from build123d import *

# Parameters (mm, degrees)
F0_R     = 12.1
F0_R_2   = 3.25
F1_DEPTH = 10
F2_R     = 11
F2_R_2   = 3.25
F3_DEPTH = 9
F4_R     = 2
F5_R     = 2


with BuildPart() as f1:
    # F0 (on Top) → F1 (new body)
    with BuildSketch(Plane.XY):
        Circle(F0_R)
        Circle(F0_R_2, mode=Mode.SUBTRACT)
    extrude(amount=F1_DEPTH)

    # F2 (on face) → F3 (cut)
    with BuildSketch(Plane.XY.offset(10)):
        Circle(F2_R)
        Circle(F2_R_2, mode=Mode.SUBTRACT)
    extrude(amount=-F3_DEPTH, mode=Mode.SUBTRACT)

    # F4
    f4_edges = [f1.edges().sort_by_distance(p)[0] for p in [
        (-12.1, 0, 0),
    ]]
    fillet(f4_edges, radius=F4_R)

    # F5
    f5_edges = [f1.edges().sort_by_distance(p)[0] for p in [
        (-11, 0, 1),
    ]]
    fillet(f5_edges, radius=F5_R)


solid = f1.part
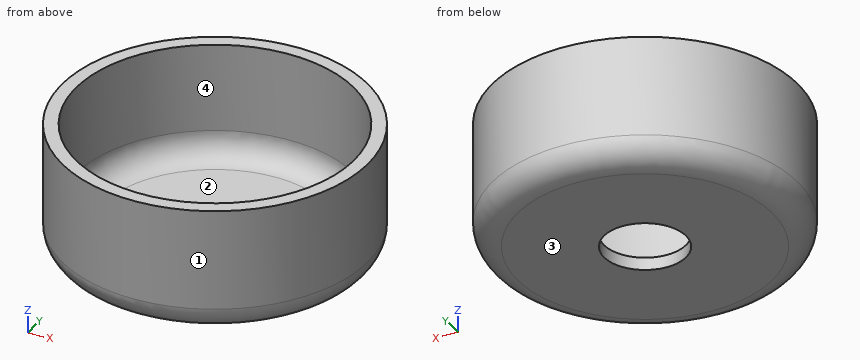
The model under review builds one solid part; all positions refer to its coordinate system, in mm. Face numbers are marked on the shaded views. Coordinates: 2 decimals unless noted, no trailing zeros. Loops run counter-clockwise (first coordinate to the right, second up) from the corner with the lowest first, then second, coordinate; pieces in that order, holes last. Notation, with made-up numbers: (-31.5, 65) -> (4.5, 65) arc R22 ccw to (4.5, 72) -> close; hole circle Ø7 at (32.5, -32.5). An arc over 180 degrees is marked (long way). Use a Markdown table: item, result. Add a question column.
1. Clearance check with flat-ended pins moving along their axes: pin 1 Ø9 at (x, y) = (-3, -1) entering from +Z; pin 2 Ø1.5 at (y, z) = (5, 4.5) entering from +X; pin 3 Ø3 at (x, z) = (8.5, 2) entering from +Y. State where each tip first meets the part, or that it passes through.
2. Add section C-C on z = 7.75. Write out the cut boundary in (x, y).
3. Draft analysis for pull direction X (two halves, no side actions). For the marked faces 1, 2, 3 and 4, state which applies: pulls with the +X half, pulls with the -X half, needs draft (parallel to the pull), parting line crosses it, or undercut.
4. Add section A-A on x = 0. Write out the cut boundary in (y, z).
5. To check wall thickness, follow line 1 (Y direction, x = 0, z = 8.75); line 2 (Z direction, x = 7.25, y = 1); line 3 (Y direction, x = 4.25, z = 7). State the ranges of each line that lie inside material, in increasing order.
Returned:
| question | item | result |
|---|---|---|
| 1 | pin 1 | stops at z = 1 |
| 1 | pin 2 | stops at x = 11.33 |
| 1 | pin 3 | stops at y = 9.87 |
| 2 | outline | circle Ø24.2 at (0, 0); hole circle Ø22 at (0, 0) |
| 3 | face 1 | parting line crosses it |
| 3 | face 2 | undercut |
| 3 | face 3 | needs draft |
| 3 | face 4 | undercut |
| 4 | outline | (-12.1, 2) arc R2 ccw to (-10.1, 0) -> (-3.25, 0) -> (-3.25, 1) -> (-9, 1) arc R2 cw to (-11, 3) -> (-11, 10) -> (-12.1, 10) -> close; (3.25, 0) -> (10.1, 0) arc R2 ccw to (12.1, 2) -> (12.1, 10) -> (11, 10) -> (11, 3) arc R2 cw to (9, 1) -> (3.25, 1) -> close |
| 5 | line 1 | y = -12.1 to -11, 11 to 12.1 |
| 5 | line 2 | z = 0 to 1 |
| 5 | line 3 | y = -11.33 to -10.15, 10.15 to 11.33 |
